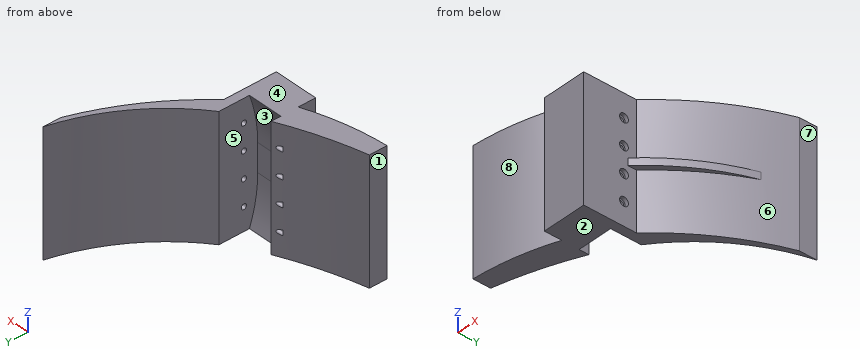
```python
from build123d import *

# Parameters (mm, degrees)
SKETCH_1_W                  = 25
SKETCH_1_H                  = 30
EXTRUDE_1_DEPTH             = 70
CUT_EXTRUDE_1_DEPTH         = 7.5
CUT_EXTRUDE_1_DEPTH_BACK    = 20
EXTRUDE_2_REACH             = 42.078
EXTRUDE_2_DIRECTION_2_REACH = 42.078
EXTRUDE_3_DEPTH             = 2
EXTRUDE_3_DEPTH_BACK        = 2
EXTRUDE_4_REACH             = 106.046
EXTRUDE_4_DIRECTION_2_REACH = 106.046
SKETCH_7_R                  = 1.5
CUT_EXTRUDE_2_DEPTH         = 30
SKETCH_8_R                  = 2.5
CUT_EXTRUDE_3_DEPTH         = 2


with BuildPart() as part:
    # 草图1 → 凸台-拉伸1 (new body)
    with BuildSketch(Plane.XY):
        Rectangle(SKETCH_1_W, SKETCH_1_H)
    extrude(amount=EXTRUDE_1_DEPTH)

    # 草图2 → 切除-拉伸1 (cut, two sides: drawn at the far end of the back side and taken through both)
    with BuildSketch(Plane(origin=(0, 0, 0), x_dir=(0, 0, -1), z_dir=(1, 0, 0)).offset(-CUT_EXTRUDE_1_DEPTH_BACK)):
        with BuildLine():
            Line((-42.9, 0), (-27.1, 0))
            ThreePointArc((-27.1, 0), (-2.605102572, 3.842268941), (19.536895265, 15))
            Line((19.536895265, 15), (-89.536895265, 15))
            ThreePointArc((-89.536895265, 15), (-67.394897428, 3.842268941), (-42.9, 0))
        make_face()
    extrude(amount=CUT_EXTRUDE_1_DEPTH + CUT_EXTRUDE_1_DEPTH_BACK, mode=Mode.SUBTRACT)

    # 凸台-拉伸2: up to this face of the body (flat: up to its plane)
    extrude_2_end = Plane(part.part.faces().sort_by_distance((0.942908229, -3.720694452, 70))[0])
    # 草图4 → 凸台-拉伸2 (add, up to the picked face)
    with BuildSketch(Plane.XY.offset(35), mode=Mode.PRIVATE) as extrude_2_sk1:
        with BuildLine():
            Line((48.883360942, 84.917683668), (48.883360942, 74.917683668))
            ThreePointArc((48.883360942, 74.917683668), (34.063250103, 42.911549159), (12.5, 15))
            Line((12.5, 15), (7.5, 15))
            Line((7.5, 15), (7.5, 22.075485157))
            ThreePointArc((7.5, 22.075485157), (33.732068033, 49.84808287), (48.883360942, 84.917683668))
        make_face()
    extrude_2_tool1 = split(extrude(extrude_2_sk1.sketch, amount=EXTRUDE_2_REACH, mode=Mode.PRIVATE), bisect_by=extrude_2_end, keep=Keep.BOTH, mode=Mode.PRIVATE)
    add(extrude_2_tool1.solids().sort_by(Axis((27.062711, 39.609343, 35), (0, 0, 1)))[0])

    # 凸台-拉伸2 direction 2: up to this face of the body (flat: up to its plane)
    extrude_2_direction_2_end = Plane(part.part.faces().sort_by_distance((0.942908229, -3.720694452, 0))[0])
    # 草图4 → 凸台-拉伸2 direction 2 (add, up to the picked face)
    with BuildSketch(Plane.XY.offset(35), mode=Mode.PRIVATE) as extrude_2_direction_2_sk1:
        with BuildLine():
            Line((48.883360942, 84.917683668), (48.883360942, 74.917683668))
            ThreePointArc((48.883360942, 74.917683668), (34.063250103, 42.911549159), (12.5, 15))
            Line((12.5, 15), (7.5, 15))
            Line((7.5, 15), (7.5, 22.075485157))
            ThreePointArc((7.5, 22.075485157), (33.732068033, 49.84808287), (48.883360942, 84.917683668))
        make_face()
    extrude_2_direction_2_tool1 = split(extrude(extrude_2_direction_2_sk1.sketch, amount=-EXTRUDE_2_DIRECTION_2_REACH, mode=Mode.PRIVATE), bisect_by=extrude_2_direction_2_end, keep=Keep.BOTH, mode=Mode.PRIVATE)
    add(extrude_2_direction_2_tool1.solids().sort_by(Axis((27.062711, 39.609343, 35), (0, 0, -1)))[0])

    # 草图5 → 凸台-拉伸3 (add, two sides: drawn at the far end of the back side and taken through both)
    with BuildSketch(Plane.XY.offset(35).offset(-EXTRUDE_3_DEPTH_BACK)):
        with BuildLine():
            Line((12.5, 15), (12.5, 10))
            ThreePointArc((12.5, 10), (30.292370974, 32.671790499), (42.5, 58.778347968))
            ThreePointArc((42.5, 58.778347968), (29.354915832, 35.618055325), (12.5, 15))
        make_face()
    extrude(amount=EXTRUDE_3_DEPTH + EXTRUDE_3_DEPTH_BACK)

    # 凸台-拉伸4: up to this face of the body (flat: up to its plane)
    extrude_4_end = Plane(part.part.faces().sort_by_distance((11.216595333, 13.322284496, 70))[0])
    # 草图6 → 凸台-拉伸4 (add, up to the picked face)
    with BuildSketch(Plane.XY.offset(35), mode=Mode.PRIVATE) as extrude_4_sk1:
        with BuildLine():
            Line((-58.137080228, -4.739738071), (-58.137080228, -14.739738071))
            ThreePointArc((-58.137080228, -14.739738071), (-34.938048555, -11.745320394), (-12.5, -5.135056795))
            Line((-12.5, -5.135056795), (-12.5, 10.260261929))
            ThreePointArc((-12.5, 10.260261929), (-34.904657371, 1.501035264), (-58.137080228, -4.739738071))
        make_face()
    extrude_4_tool1 = split(extrude(extrude_4_sk1.sketch, amount=EXTRUDE_4_REACH, mode=Mode.PRIVATE), bisect_by=extrude_4_end, keep=Keep.BOTH, mode=Mode.PRIVATE)
    add(extrude_4_tool1.solids().sort_by(Axis((-33.740556, -4.265759, 35), (0, 0, 1)))[0])

    # 凸台-拉伸4 direction 2: up to this face of the body (flat: up to its plane)
    extrude_4_direction_2_end = Plane(part.part.faces().sort_by_distance((11.216595333, 13.322284496, 0))[0])
    # 草图6 → 凸台-拉伸4 direction 2 (add, up to the picked face)
    with BuildSketch(Plane.XY.offset(35), mode=Mode.PRIVATE) as extrude_4_direction_2_sk1:
        with BuildLine():
            Line((-58.137080228, -4.739738071), (-58.137080228, -14.739738071))
            ThreePointArc((-58.137080228, -14.739738071), (-34.938048555, -11.745320394), (-12.5, -5.135056795))
            Line((-12.5, -5.135056795), (-12.5, 10.260261929))
            ThreePointArc((-12.5, 10.260261929), (-34.904657371, 1.501035264), (-58.137080228, -4.739738071))
        make_face()
    extrude_4_direction_2_tool1 = split(extrude(extrude_4_direction_2_sk1.sketch, amount=-EXTRUDE_4_DIRECTION_2_REACH, mode=Mode.PRIVATE), bisect_by=extrude_4_direction_2_end, keep=Keep.BOTH, mode=Mode.PRIVATE)
    add(extrude_4_direction_2_tool1.solids().sort_by(Axis((-33.740556, -4.265759, 35), (0, 0, -1)))[0])

    # 草图7 → 切除-拉伸2 (cut)
    with BuildSketch(Plane(origin=(12.5, 0, 0), x_dir=(0, 0, -1), z_dir=(1, 0, 0))):
        with Locations(Location((-27.684621138, 7.856985716, 0), (0, 0, 7.606747505))):
            Circle(SKETCH_7_R)
        with Locations(Location((-42.315378862, 7.856985716, 0), (0, 0, 7.606747505))):
            Circle(SKETCH_7_R)
        with Locations(Location((-56.946136586, 7.856985716, 0), (0, 0, 7.606747505))):
            Circle(SKETCH_7_R)
        with Locations(Location((-13.053863414, 7.856985716, 0), (0, 0, 7.606747505))):
            Circle(SKETCH_7_R)
    extrude(amount=-CUT_EXTRUDE_2_DEPTH, mode=Mode.SUBTRACT)

    # 草图8 → 切除-拉伸3 (cut)
    with BuildSketch(Plane(origin=(12.5, 0, 0), x_dir=(0, 0, -1), z_dir=(1, 0, 0))):
        with Locations((-56.946136586, 7.856985716)):
            Circle(SKETCH_8_R)
        with Locations((-42.315378862, 7.856985716)):
            Circle(SKETCH_8_R)
        with Locations((-27.684621138, 7.856985716)):
            Circle(SKETCH_8_R)
        with Locations((-13.053863414, 7.856985716)):
            Circle(SKETCH_8_R)
    extrude(amount=-CUT_EXTRUDE_3_DEPTH, mode=Mode.SUBTRACT)


solid = part.part
```
Here's how the part is built. I have some questions about the finished solid (model axes, mm). Face numbers are marked on the shaded views. A direction names the side the tool comes from. Give positions to 0.01 mm unless a question says otherwise; leave off trailing zeros. Order: outer loops, then holes, each group sorted by start corner. A loop starts at its lowest first (then second) coordinate and runs counter-clockwise, first axis right, second up. Notation, with made-up numbers: M 9,-32 L 42,-32 A21 ccw 42,2 Z; hole C 70,52.5 d3. An arc over 180 degrees is marked long. Use a Markdown table: item, result. Add a question column.
1. For pin 1 Ø8 at (x, z) = (-32, 27.5) entering from +Y; pin 2 Ø4 at (y, z) = (7.86, 13.05) entering from +X; pin 3 Ø8 at (x, z) = (-34.5, 49) entering from -Y, each with a flat end and sliding along its axis, tell me the tip position at first contact or that it passes through.
2. On a 3-axis mill with a long thin cutter (end or side, diameter ignored), from which of +Z, -Z, +X, -X, +Y, -Y can I reach the whole of each face in a straight line? I mean the marked faces 5, 6, 7 and 8. Say none if no direction works.
3. Suppose I cut it at B-B (x = 24.5). List the corners of the cut face in (y, z) for me.
4. Suppose I cut it at C-C (z = 9). List the corners of the cut face in (x, y) for me.
5. I need wall thicknesses on probe 1 along Y at (x, z) = (24.5, 39); probe 2 along X at (y, z) = (39, 10); probe 3 along X at (y, z) = (37, 20.5). Which ranges of each line are inside material? Lowest first, please. Write a range as from..to.
6. Suppose I cut it at A-A (y = 1.5). List the corners of the cut face in (x, z) for me, and give its area (3 significant figures).
7. If we mould it in two halves opening along Z, with no side actions, what happens to the marked faces 1, 2, 3 and 4? For each: +Z half, -Z half, draft (parallel to the pull), parting line (faces both ways), or undercut.
8. Suppose I cut it at D-D (y = 27). List the corners of the cut face in (x, z) for me.
Results list:
| question | item | result |
|---|---|---|
| 1 | pin 1 | stops at y = 3.9 |
| 1 | pin 2 | stops at x = 10.5 |
| 1 | pin 3 | stops at y = -12.45 |
| 2 | face 5 | +Y |
| 2 | face 6 | +X, -Y |
| 2 | face 7 | +Z, -Z, +X, +Y, -Y |
| 2 | face 8 | +Z, -Z, -Y |
| 3 | outline | M 24.06,33 L 28.92,33 L 28.92,0 L 37.74,0 L 37.74,70 L 28.92,70 L 28.92,37 L 24.06,37 Z |
| 4 | outline | M -58.14,-14.74 A148.08 ccw -12.5,-5.14 L -12.5,-15 L 12.5,-15 L 12.5,15 A157.69 ccw 48.88,74.92 L 48.88,84.92 A110 cw 7.5,22.08 L 7.5,2.07 L -12.5,2.07 L -12.5,10.26 A218.29 cw -58.14,-4.74 Z |
| 5 | probe 1 | y = 28.92..37.74 |
| 5 | probe 2 | x = 25.59..31.61 |
| 5 | probe 3 | x = 23.84..30.29 |
| 6 | outline | M -34.91,0 L 12.5,0 L 12.5,70 L -34.91,70 Z; hole M -12.5,11.68 L 7.5,11.68 L 7.5,58.32 L -12.5,58.32 Z |
| 6 | area | 2,390 mm² |
| 7 | face 1 | draft |
| 7 | face 2 | -Z half |
| 7 | face 3 | undercut |
| 7 | face 4 | +Z half |
| 8 | outline | M 13.65,0 L 23.01,0 L 23.01,33 L 26.59,33 L 26.59,37 L 23.01,37 L 23.01,70 L 13.65,70 Z |
